```python
from build123d import *

# Parameters (mm, degrees)
RECTANGULAR_TUBE_3_X_2_X_0_25_1_DEPTH = 498.475
CUT_EXTRUDE1_DEPTH                    = 254.408960785


with BuildPart() as part:
    # Sketch13 → Rectangular tube 3 X 2 X 0.25(1) (new body)
    with BuildSketch(Plane.ZY.offset(-249.2375)):
        with BuildLine():
            Line((-7.9375, -38.1), (7.9375, -38.1))
            ThreePointArc((7.9375, -38.1), (11.305096045, -36.705096045), (12.7, -33.3375))
            Line((12.7, -33.3375), (12.7, 33.3375))
            ThreePointArc((12.7, 33.3375), (11.305096045, 36.705096045), (7.9375, 38.1))
            Line((7.9375, 38.1), (-7.9375, 38.1))
            ThreePointArc((-7.9375, 38.1), (-11.305096045, 36.705096045), (-12.7, 33.3375))
            Line((-12.7, 33.3375), (-12.7, -33.3375))
            ThreePointArc((-12.7, -33.3375), (-11.305096045, -36.705096045), (-7.9375, -38.1))
        make_face()
        with BuildLine():
            Line((-7.9375, -35.052), (7.9375, -35.052))
            ThreePointArc((7.9375, -35.052), (9.149834576, -34.549834576), (9.652, -33.3375))
            Line((9.652, -33.3375), (9.652, 33.3375))
            ThreePointArc((9.652, 33.3375), (9.149834576, 34.549834576), (7.9375, 35.052))
            Line((7.9375, 35.052), (-7.9375, 35.052))
            ThreePointArc((-7.9375, 35.052), (-9.149834576, 34.549834576), (-9.652, 33.3375))
            Line((-9.652, 33.3375), (-9.652, -33.3375))
            ThreePointArc((-9.652, -33.3375), (-9.149834576, -34.549834576), (-7.9375, -35.052))
        make_face(mode=Mode.SUBTRACT)
    extrude(amount=RECTANGULAR_TUBE_3_X_2_X_0_25_1_DEPTH)

    # s → Cut-Extrude1 (cut, through all)
    with BuildSketch(Plane.XY.offset(12.7)):
        Polygon((-249.2375, -38.1), (-249.2375, 38.1), (-82.031860485, 38.1), align=None)
    extrude(amount=-CUT_EXTRUDE1_DEPTH, mode=Mode.SUBTRACT)


solid = part.part
```
The model under review builds one solid part; all positions refer to its coordinate system, in mm. A direction names the side the tool comes from. Round coordinates to 2 decimals unless told otherwise and drop trailing zeros. Loops run counter-clockwise (first coordinate to the right, second up) from the corner with the lowest first, then second, coordinate; pieces in that order, holes last. Notation, with made-up numbers: (78, 88.25) -> (113, 88.25) arc R12 cw to (113, 110.25) -> close; hole circle Ø8 at (-28.5, 7.25). An arc over 180 degrees is marked (long way). Answer in a Markdown table with one row per item.
1) Consider section A-A, the plane x = 95.5. Write out the cut boundary in (y, z) (1 decimal), plus the area to 3 significant figures.
Taken from the geometry:
| item | result |
|---|---|
| outline | (-38.1, -7.9) arc R4.8 ccw to (-33.3, -12.7) -> (33.3, -12.7) arc R4.8 ccw to (38.1, -7.9) -> (38.1, 7.9) arc R4.8 ccw to (33.3, 12.7) -> (-33.3, 12.7) arc R4.8 ccw to (-38.1, 7.9) -> close; hole (-35.1, -7.9) arc R1.7 ccw to (-33.3, -9.7) -> (33.3, -9.7) arc R1.7 ccw to (35.1, -7.9) -> (35.1, 7.9) arc R1.7 ccw to (33.3, 9.7) -> (-33.3, 9.7) arc R1.7 ccw to (-35.1, 7.9) -> close |
| area | 565 mm² |
2) Tool access review of faces 5 (the flat face through (-165.2, 0.2, -10.3)), 6 (the flat face through (7, -35.052, 0)): name each direction out of +Z, -Z, +X, -X, +Y, -Y from which nothing blocks a thin tool from reaching the whole face with its end or side.
Taken from the geometry:
| item | result |
|---|---|
| face 5 | +Z, -Z, -X, +Y |
| face 6 | +X, -X |
3) Consider section B-B, the plane z = -2.5. Write out the cut boundary in (x, y), plus the area to 3 significant figures.
Taken from the geometry:
| item | result |
|---|---|
| outline | (-249.24, -38.1) -> (249.24, -38.1) -> (249.24, -35.05) -> (-242.55, -35.05) -> close; (-88.72, 35.05) -> (249.24, 35.05) -> (249.24, 38.1) -> (-82.03, 38.1) -> close |
| area | 2,530 mm² |
4) Draft analysis for pull direction Y (two halves, no side actions). For faces 1 (the flat face through (63, 0, -9.652)), 2 (the flat face through (63, 0, -12.7)), 3 (the flat face through (63, 0, 9.652)), 4 (the flat face through (86, 38.1, 0)), state which applies: pulls with the +Y half, pulls with the -Y half, needs draft (parallel to the pull), parting line crosses it, or undercut.
Taken from the geometry:
| item | result |
|---|---|
| face 1 | undercut |
| face 2 | needs draft |
| face 3 | undercut |
| face 4 | pulls with the +Y half |
5) Consider section C-C, the plane y = 21.5. Write out the cut boundary in (x, z).
Taken from the geometry:
| item | result |
|---|---|
| outline | (-118.46, -12.7) -> (249.24, -12.7) -> (249.24, -9.65) -> (-118.46, -9.65) -> close; (-118.46, 9.65) -> (249.24, 9.65) -> (249.24, 12.7) -> (-118.46, 12.7) -> close |
6) Consider section D-D, the plane x = -131. Write out the cut boundary in (y, z) (1 decimal).
Taken from the geometry:
| item | result |
|---|---|
| outline | (-38.1, -7.9) arc R4.8 ccw to (-33.3, -12.7) -> (15.8, -12.7) -> (15.8, -9.7) -> (-33.3, -9.7) arc R1.7 cw to (-35.1, -7.9) -> (-35.1, 7.9) arc R1.7 cw to (-33.3, 9.7) -> (15.8, 9.7) -> (15.8, 12.7) -> (-33.3, 12.7) arc R4.8 ccw to (-38.1, 7.9) -> close |
7) Wall thickness on line 1 along Y through (x, z) = (-77.5, 4.5); line 2 along Z through (x, y) = (92.5, -27.5); line 3 along Y through (x, z) = (209.5, 8.5): over which ranges is each line inside the solid? List them lowest first.
Taken from the geometry:
| item | result |
|---|---|
| line 1 | y = -38.1 to -35.05, 35.05 to 38.1 |
| line 2 | z = -12.7 to -9.65, 9.65 to 12.7 |
| line 3 | y = -38.07 to -34.96, 34.96 to 38.07 |
